Geometry check sheet. Reference: the model listing, model coordinates, mm. A direction names the side the tool comes from. Give positions to 0.01 mm unless a question says otherwise; leave off trailing zeros. Write each loop counter-clockwise with the first axis right and the second up, starting at its lowest first coordinate (ties: lowest second). Pieces come first, ordered by that corner, then holes. Notation, with made-up numbers: (21.25, 5) -> (40.25, 5) arc R21 cw to (40.25, 11) -> close; hole circle Ø5 at (-9.75, 79.25). An arc over 180 degrees is marked (long way). One line per item, written item: value.
Autodesk Inventor part; units mm, degrees
ref_plane "YZ Plane" through (0, 0, 0) normal (1, 0, 0) x (0, 1, 0)
ref_plane "XZ Plane" through (0, 0, 0) normal (0, 1, 0) x (-1, 0, 0)
ref_plane "XY Plane" through (0, 0, 0) normal (0, 0, 1) x (1, 0, 0)
sketch "Esquisse1" plane through (0, 0, 0) normal (1, 0, 0) x (0, 1, 0)
  line L0 (0, 0) -> (0, 42.75) construction
  line L1 (98.5, -2.5) -> (102.5, -2.5)
  line L2 (102.5, -2.5) -> (102.5, 0)
  line L3 (102.5, 0) -> (111, 0)
  line L4 (111, 0) -> (111, 4.6)
  line L5 (111, 4.6) -> (102, 4.6)
  line L6 (102, 4.6) -> (99.0675, 15.5441)
  arc A0 (99.0675, 15.5441) -> (94.2379, 19.25) centre (94.2379, 14.25) ccw
  line L7 (94.2379, 19.25) -> (40, 19.25)
  line L8 (15, 39.25) -> (16.5, 39.25)
  line L9 (16.5, 39.25) -> (17.5, 38.25)
  line L10 (17.5, 38.25) -> (17.5, 27.25)
  line L11 (17.5, 27.25) -> (16.5, 27.25)
  line L12 (16.5, 27.25) -> (16.5, 25.25)
  line L13 (16.5, 25.25) -> (34, 25.25)
  line L14 (34, 25.25) -> (35, 24.25)
  arc A1 (35, 24.25) -> (40, 19.25) centre (40, 24.25) ccw
  line L15 (94.6398, 14.75) -> (34.5, 14.75)
  line L16 (98.3296, 6.7069) -> (96.5717, 13.2676)
  arc A2 (96.5717, 13.2676) -> (94.6398, 14.75) centre (94.6398, 12.75) ccw
  line L17 (98.5, -2.5) -> (98.5, 5.4128)
  arc A3 (98.5, 5.4128) -> (98.3296, 6.7069) centre (93.5, 5.4128) ccw
  line L18 (29.5, 9.75) -> (29.5, 8.25)
  arc A4 (34.5, 14.75) -> (29.5, 9.75) centre (34.5, 9.75) ccw
  line L19 (29.5, 8.25) -> (22, 8.25)
  line L20 (22, 8.25) -> (22, 20.25)
  line L21 (22, 20.25) -> (18.5, 20.25)
  line L22 (18.5, 20.25) -> (18.5, 21.25)
  line L23 (18.5, 21.25) -> (11.7, 26.95)
  line L24 (11.7, 26.95) -> (11.7, 32.25)
  line L25 (11.7, 32.25) -> (15, 32.25)
  line L26 (15, 32.25) -> (15, 39.25)
  line L27 (40, 24.25) -> (35, 24.25) construction
  dimension "d0" = 111
  dimension "d1" = 102.5
  dimension "d3" = 2.5
  dimension "d4" = 4.6
  dimension "d5" = 0.5
  dimension "d8" = 5
  dimension "d16" = 105
  dimension "d17" = 42.75
  dimension "d40" = 39.25
  dimension "d42" = 1
  dimension "d43" = 1
  dimension "d45" = 1
  dimension "d46" = 2
  dimension "d47" = 1
  dimension "d48" = 1
  dimension "d49" = 5
  dimension "d50" = 17.5
  dimension "d51" = 35
  dimension "d56" = 23.5
  dimension "d57" = 3
  dimension "d58" = 4.5
  dimension "d59" = 2
  dimension "d60" = 98.5
  dimension "d61" = 5
  dimension "d62" = 5
  dimension "d63" = 22
  dimension "d64" = 29.5
  dimension "d65" = 17
  dimension "d66" = 12
  dimension "d67" = 18.5
  dimension "d68" = 1
  dimension "d69" = 5.7
  dimension "d70" = 6.8
  dimension "d71" = 7
  dimension "d72" = 15
revolve "Révolution1" add sketch "Esquisse1" angle 360 about axis through (0, 0, 0) along (0, 0, 1)
sketch "Esquisse2" plane through (0, 0, 4.6) normal (0, 0, 1) x (1, 0, 0)
  circle A0 centre (-106, 0) radius 2.65
  circle A1 centre (-74.9533, 74.9533) radius 2.65
  circle A2 centre (0, 106) radius 2.65
  circle A3 centre (74.9533, 74.9533) radius 2.65
  circle A4 centre (106, 0) radius 2.65
  circle A5 centre (74.9533, -74.9533) radius 2.65
  circle A6 centre (0, -106) radius 2.65
  circle A7 centre (-74.9533, -74.9533) radius 2.65
  line L0 (0, 0) -> (-106, 0) construction
  dimension "d19" = 5.3
  dimension "d22" = 360
  dimension "d24" = 212
extrude "Extrusion1" cut sketch "Esquisse2" against normal through all
thread "Filetage1"
thread "Filetage2"
properties part number "Flasque 1"
1) Sectioned sample at C-C on x = 0. Give the number of separate pieces and of enclosed holes in the cut face, plus the area to 3 significant figures.
Verdict:
separate pieces: 4
enclosed holes: 0
area: 1,270 mm^2
2) Scan lines: probe 1 along Y at (x, z) = (0, 2); probe 2 along Y at (x, z) = (10, 14); probe 3 along X at (y, z) = (0, 35.5). Record each from-to range of solid material in increasing order.
Verdict:
probe 1: -111 to -108.65, -103.35 to -98.5, 98.5 to 103.35, 108.65 to 111
probe 2: -98.98 to -95.68, -30.26 to -19.6, 19.6 to 30.26, 95.68 to 98.98
probe 3: -17.5 to -15, 15 to 17.5
3) Sectioned sample at A-A on x = 106. Record the cut outline in (y, z).
Verdict:
outline: (-32.94, 0) -> (-2.65, 0) -> (-2.65, 4.6) -> (-32.94, 4.6) -> close; (2.65, 0) -> (32.94, 0) -> (32.94, 4.6) -> (2.65, 4.6) -> close
4) Mould release check, pull along Z, two halves, no side actions. Record for faces 1 (the cylindrical face through (-0.57, -108.59, 2.33)), 2 (the conical face through (-96.89, -21.52, 14.86)), 3 (the cylindrical face through (-6.32, 15.24, 26.24)): released by +Z, released by -Z, zero draft, split by the parting line, or undercut.
Verdict:
face 1: zero draft
face 2: released by +Z
face 3: undercut
5) Depth check by flat-ended pin: pin 1 Ø6 at (y, z) = (-12, 16) entering from +X; pin 2 Ø10 at (x, y) = (-68.5, -44.5) entering from +Z; pin 3 Ø5 at (x, y) = (49.5, -14.5) entering from -Z. Enter the tip coordinate at first touch or a pass-through.
Verdict:
pin 1: x = 99.1
pin 2: z = 19.25
pin 3: z = 14.75
6) Tool access check on faces 4 (the flat face through (90, 49, 4.6)), 5 (the flat face through (-1, 41, 14.75)), 6 (the flat face through (-5, -16, 27.25)). Record the directions out of +Z, -Z, +X, -X, +Y, -Y that give a thin tool (end or side, any length) a straight path to the whole face; none if there is none.
Verdict:
face 4: +Z
face 5: -Z
face 6: none
